For this review, use the dimensioned drawing (mm, ordinates from the lowest corner) and the shaded views. Round coordinates to 2 decimals unless told otherwise and drop trailing zeros. Loops run counter-clockwise (first coordinate to the right, second up) from the corner with the lowest first, then second, coordinate; pieces in that order, holes last. Notation, with made-up numbers: M 87,-5.5 L 116,-5.5 A18 cw 116,-1.5 Z; hole C -3,14 d11. An arc over 180 degrees is marked long. Answer as a JSON object with one key per item and string values. Group by question number.
Item 1: Consider section B-B (z = 295). Give the boundary of the cut face in (x, y), and give its area (3 significant figures).
Item 2: To check wall thickness, follow line 1 (Y direction, x = 2.5, z = 391); line 2 (Z direction, x = 2.75, y = 64.5); line 3 (X direction, y = 18.5, z = 366). State the ranges of each line that lie inside material, in increasing order.
Item 3: Consider section C-C (y = 71.5). Give the boundary of the cut face in (x, z).
Item 4: Insertion check: P1, Ø6.5, axis at x = 4, y = 93.5, coming from the +Z side; P2, Ø4, axis at x = 8, y = 68, coming from the -Z side; P3, Ø4, axis at x = 3.5, z = 524, coming from the +Y side. Each pin has a flat end and moves straight along its axis. Give the tip position at first contact, or say it passes through.
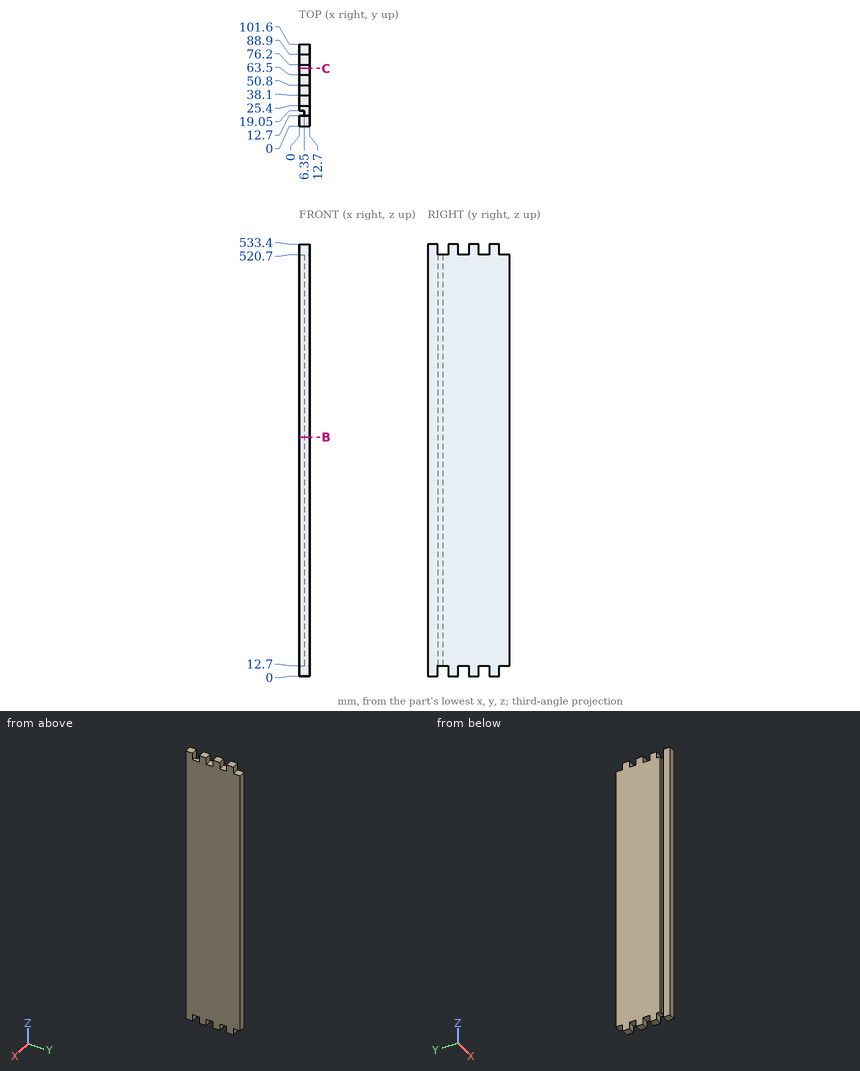
Geometry results:
{
 "1": {"outline": "M 0,0 L 12.7,0 L 12.7,101.6 L 0,101.6 L 0,19.05 L 6.35,19.05 L 6.35,12.7 L 0,12.7 Z", "area": "1,250 mm^2"},
 "2": {"line 1": "y = 0 to 12.7, 19.05 to 101.6", "line 2": "z = 12.7 to 520.7", "line 3": "x = 6.35 to 12.7"},
 "3": {"outline": "M 0,12.7 L 12.7,12.7 L 12.7,520.7 L 0,520.7 Z"},
 "4": {"P1": "stops at z = 520.7", "P2": "stops at z = 12.7", "P3": "stops at y = 88.9"}
}
